Autodesk Inventor part; units mm, degrees
ref_plane "YZ Plane" through (0, 0, 0) normal (1, 0, 0) x (0, 1, 0)
ref_plane "XZ Plane" through (0, 0, 0) normal (0, 1, 0) x (-1, 0, 0)
ref_plane "XY Plane" through (0, 0, 0) normal (0, 0, 1) x (1, 0, 0)
sketch "Sketch1" plane through (0, 0, 0) normal (0, 1, 0) x (-1, 0, 0)
  line L0 (0, 0) -> (-149.86, 0)
  line L1 (-149.86, 0) -> (-149.86, -50.8)
  line L2 (-149.86, -50.8) -> (0, -50.8)
  line L3 (0, -50.8) -> (0, 0)
  circle A0 centre (-43.942, -25.4) radius 12.7
  circle A1 centre (-29.972, -39.37) radius 1.5875
  circle A2 centre (-57.912, -39.37) radius 1.5875
  circle A3 centre (-57.912, -11.43) radius 1.5875
  circle A4 centre (-29.972, -11.43) radius 1.5875
  line L4 (-74.93, -50.8) -> (-74.93, 0) construction
  circle A5 centre (-5.588, -44.704) radius 2.3495
  circle A6 centre (-5.588, -25.4) radius 2.3495
  circle A7 centre (-5.588, -6.096) radius 2.3495
  circle A8 centre (-105.918, -25.4) radius 12.7
  circle A9 centre (-119.888, -39.37) radius 1.5875
  circle A10 centre (-91.948, -39.37) radius 1.5875
  circle A11 centre (-91.948, -11.43) radius 1.5875
  circle A12 centre (-119.888, -11.43) radius 1.5875
  circle A13 centre (-144.272, -44.704) radius 2.3495
  circle A14 centre (-144.272, -25.4) radius 2.3495
  circle A15 centre (-144.272, -6.096) radius 2.3495
  point P0 (-74.93, -25.4)
  dimension "d0" = 149.86
  dimension "d1" = 50.8
  dimension "d2" = 30.988
  dimension "d3" = 25.4
  dimension "d4" = 25.4
  dimension "d5" = 13.97
  dimension "d6" = 13.97
  dimension "d7" = 13.97
  dimension "d8" = 13.97
  dimension "d9" = 13.97
  dimension "d10" = 13.97
  dimension "d11" = 13.97
  dimension "d12" = 13.97
  dimension "d13" = 3.175
  dimension "d14" = 3.175
  dimension "d15" = 3.175
  dimension "d16" = 3.175
  dimension "d17" = 5.588
  dimension "d18" = 6.096
  dimension "d19" = 5.588
  dimension "d20" = 25.4
  dimension "d21" = 6.096
  dimension "d22" = 5.588
  dimension "d23" = 4.699
  dimension "d24" = 4.699
  dimension "d25" = 4.699
extrude "Extrusion1" add sketch "Sketch1" along normal blind 3.175
properties part number "3D Camera Mount 3"
Part model, mm, in its own coordinate system. Coordinates: 2 decimals unless noted, no trailing zeros. Loops run counter-clockwise (first coordinate to the right, second up) from the corner with the lowest first, then second, coordinate; pieces in that order, holes last. Notation, with made-up numbers: (-1, -26.5) - (36, -26.5) arc R22 ccw to (36, 5.5) - close; hole circle Ø6 at (22.25, -8.75). An arc over 180 degrees is marked (long way). Write item = value, one per line. Start each with the question number.
Item 1: Cut at D-D, the plane z = -17. Give the cut face in (x, y) (3 decimals).
Item 2: Cut at C-C, the plane y = 1.55. State how many separate pieces and enclosed holes the cut face has, and give its area (3 significant figures).
Item 3: Mould opens along X. For faces 1 (the flat face through (76, 0, -25)), 2 (the cylindrical face through (57.06, 1.57, -40.71)) say: released by +X, released by -X, zero draft, split by the parting line, or undercut.
Item 4: Cut at B-B, the plane x = 49. Give the cut face in (y, z) (3 decimals), and give its area (3 significant figures).
Item 5: Wall check: L1, parallel to X at y = 2.95, z = -22.5; L2, parallel to X at y = 2, z = -39.5; L3, parallel to Z at x = 142.5, y = 1. Give the ranges that are in metal, low to high. Write a range as from..to.
Item 6: Cut at A-A, the plane z = -11.43. Give the cut face in (x, y) (1 decimal).
The answers:
q1.outline = (0, 0) - (34.417, 0) - (34.417, 3.175) - (0, 3.175) - close; (53.467, 0) - (96.393, 0) - (96.393, 3.175) - (53.467, 3.175) - close; (115.443, 0) - (149.86, 0) - (149.86, 3.175) - (115.443, 3.175) - close
q2.separate_pieces = 1
q2.enclosed_holes = 16
q2.area = 6,430 mm2
q3.face_1 = zero draft
q3.face_2 = undercut
q4.outline = (0, -50.8) - (3.175, -50.8) - (3.175, -37.049) - (0, -37.049) - close; (0, -13.751) - (3.175, -13.751) - (3.175, 0) - (0, 0) - close
q4.area = 87.3 mm2
q5.L1 = 0..31.58, 56.31..93.55, 118.28..149.86
q5.L2 = 0..28.39, 31.55..56.33, 59.49..90.37, 93.53..118.31, 121.47..149.86
q5.L3 = -50.8..-46.25, -43.16..-26.94, -23.86..-7.64, -4.55..0
q6.outline = (0, 0) - (28.4, 0) - (28.4, 3.2) - (0, 3.2) - close; (31.6, 0) - (56.3, 0) - (56.3, 3.2) - (31.6, 3.2) - close; (59.5, 0) - (90.4, 0) - (90.4, 3.2) - (59.5, 3.2) - close; (93.5, 0) - (118.3, 0) - (118.3, 3.2) - (93.5, 3.2) - close; (121.5, 0) - (149.9, 0) - (149.9, 3.2) - (121.5, 3.2) - close
